Source: CAD feature listing. Evaluate the final solid. Frame: model axes, mm. Face numbers are marked on the shaded views. A direction names the side the tool comes from. Round coordinates to 2 decimals unless told otherwise and drop trailing zeros. Loops run counter-clockwise (first coordinate to the right, second up) from the corner with the lowest first, then second, coordinate; pieces in that order, holes last. Notation, with made-up numbers: (-6.75, 47.25) -> (22.25, 47.25) arc R26 ccw to (22.25, 81.25) -> close; hole circle Ø4 at (-2.75, 88). An arc over 180 degrees is marked (long way). Write item = value, one per line.
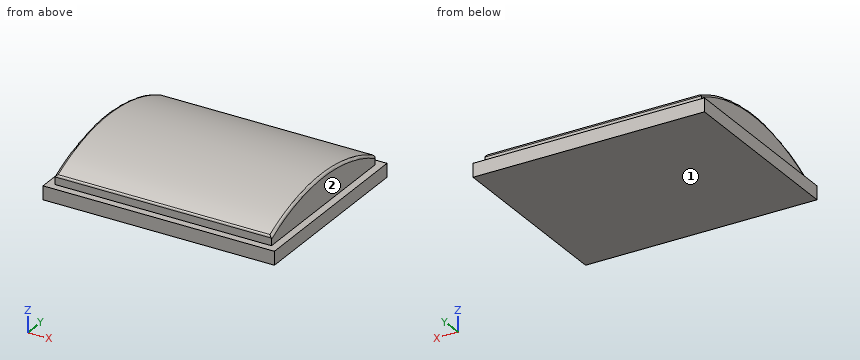
Autodesk Inventor part; units mm, degrees
ref_plane "Work Plane1" through (0, 0, 18) normal (0, 0, -1) x (-1, 0, 0)
ref_plane "YZ Plane" through (0, 0, 0) normal (1, 0, 0) x (0, 1, 0)
ref_plane "XZ Plane" through (0, 0, 0) normal (0, 1, 0) x (-1, 0, 0)
sketch "Sketch1" plane through (0, 0, 0) normal (0, 0, 1) x (1, 0, 0)
  line L0 (0, 0) -> (94, 0)
  line L1 (94, 0) -> (94, 76)
  line L2 (94, 76) -> (0, 76)
  line L3 (0, 76) -> (0, 0)
  line L4 (4.75, 10.5) -> (89.25, 10.5)
  line L5 (89.25, 10.5) -> (89.25, 65.5)
  line L6 (89.25, 65.5) -> (4.75, 65.5)
  line L7 (4.75, 65.5) -> (4.75, 10.5)
  dimension "d0" = 84.5
  dimension "d1" = 55
  dimension "d2" = 76
  dimension "d3" = 94
  dimension "d4" = 10.5
  dimension "d5" = 4.75
  dimension "d6" = 4.75
  dimension "d7" = 10.5
extrude "Extrusion1" add sketch "Sketch1" along normal blind 17.5 contours L3 L2 L1 L0 | L7 L6 L5 L4
ref_plane "Work Plane1" through (0, 0, 18) normal (0, 0, -1) x (-1, 0, 0)
sketch "Sketch3" plane through (0, 0, 18) normal (0, 0, -1) x (-1, 0, 0)
  line L0 (0, 0) -> (-94, 0)
  line L1 (0, 76) -> (-3, 76)
  line L2 (-3, 76) -> (-3, 0)
  line L3 (-3, 0) -> (0, 0)
  line L4 (0, 0) -> (0, 76)
  line L5 (-94, 0) -> (-91, 0)
  line L6 (-91, 0) -> (-91, 76)
  line L7 (-91, 76) -> (-94, 76)
  line L8 (-94, 76) -> (-94, 0)
  line L9 (-94, 76) -> (0, 76)
  dimension "d16" = 3
  dimension "d17" = 3
  dimension "d32" = 0
extrude "Extrusion3" cut sketch "Sketch3" along normal blind 12.5 contours L0 L2 L1 L4 | L0 L8 L7 L6
sketch "Sketch4" plane through (0, 0, 18) normal (0, 0, -1) x (-1, 0, 0)
  line L0 (0, 76) -> (0, 0)
  line L1 (-94, 76) -> (-94, 0)
  line L2 (0, 76) -> (-94, 76)
  line L3 (-94, 76) -> (-94, 73)
  line L4 (-94, 73) -> (0, 73)
  line L5 (0, 73) -> (0, 76)
  line L6 (-104.5, 0) -> (0, 0)
  line L7 (0, 0) -> (-94, 0)
  line L8 (-94, 0) -> (-94, 3)
  line L9 (-94, 3) -> (0, 3)
  line L10 (0, 3) -> (0, 0)
  point P0 (-104.5, 75.9892)
  point P1 (-104.5, 3.0108)
  point P2 (0, 3)
  point P3 (-94, 3)
  point P4 (-94, 3)
  point P5 (-94, 0)
  point P6 (-104.5, 75.9892)
  point P7 (-95, 6)
  dimension "d20" = 3
  dimension "d21" = 3
extrude "Extrusion4" cut sketch "Sketch4" along normal blind 12.5 contours L0 L4 L1 L2 | L0 L6 L1 L9
sketch "Sketch5" plane through (94, 0, 0) normal (1, 0, 0) x (0, 0, -1)
  line L0 (-17.5, 3) -> (-17.5, 73)
  line L1 (0, 76) -> (-5.5, 76)
  line L2 (0, 0) -> (-5.5, 0)
  arc A0 (-7.5, 76) -> (-7.5, 0) centre (59.7, 38) ccw
  line L3 (0, 0) -> (0, 76)
  line L4 (-17.5, 38) -> (-17.5, 3)
  line L5 (-17.5, 3) -> (-5.5, 3)
  line L6 (-9.1102, 3) -> (-17.5, 3)
  line L7 (-5.5, 73) -> (-17.5, 73)
  line L8 (-9.1102, 73) -> (-17.5, 73)
  line L9 (-17.5, 73) -> (-17.5, 38)
  point P0 (-15, 3)
  point P1 (-15, 73)
  point P2 (-15, 73)
  point P3 (-15, 3)
  dimension "d24" = 38
  dimension "d25" = 38
  dimension "d26" = 7.5
  dimension "d27" = 7.5
extrude "Extrusion5" cut sketch "Sketch5" against normal through all
fillet "Fillet1" radius 1 4 edges at (47, 73, 9.1102) (91, 38, 17.5) (3, 38, 17.5) (47, 3, 9.1102)
equation "\"d17\" = d16"
equation "\"d21\" = d20"
equation "\"d27\" = d26"
properties part number "MainHousing_Screen Acrylic"
1. Set-up query: the marked faces 1 and 2. Return all of +Z, -Z, +X, -X, +Y, -Y with unobstructed straight access to the full face (end or side cutting, diameter ignored); none if empty.
Evaluation:
face_1 = -Z, +X, -X, +Y, -Y
face_2 = +Z, +X, +Y, -Y
2. Contact query for flat-ended pins moving along their axis: pin 1 Ø3.5 at (x, z) = (37.5, 7) entering from -Y; pin 2 Ø1 at (x, y) = (31, 13) entering from +Z; pin 3 Ø10 at (x, y) = (78.5, 40) entering from +Z; pin 4 Ø0.9 at (x, z) = (45, 6.5) entering from +Y. Output: stop coordinate, or through.
Evaluation:
pin_1 = 0
pin_2 = 13.51
pin_3 = 17.5
pin_4 = 73
3. Section query A-A (x = 85.5). Return the cut outline in (y, z), then the cut area to 3 significant figures.
Evaluation:
outline = (0, 0) -> (76, 0) -> (76, 5.5) -> (73, 5.5) -> (73, 8.49) arc R1 ccw to (72.45, 9.39) arc R77.2 ccw to (3.55, 9.39) arc R1 ccw to (3, 8.49) -> (3, 5.5) -> (0, 5.5) -> close
area = 1,070 mm²
4. Line query: probe 1 along Y at (x, z) = (25, 8.5); probe 2 along X at (y, z) = (34, 9); probe 3 along Z at (x, y) = (16.5, 20.5). Output: solid intervals per line, ascending. Write a range as from..to.
Evaluation:
probe_1 = 3..73
probe_2 = 3..91
probe_3 = 0..15.49
